Answer from the drawing. Dimensions are ordinates in mm from the lowest x, y and z of the part. Give positions to 0.01 mm unless a question says otherwise; leave off trailing zeros. Write each loop counter-clockwise with the first axis right and the second up, starting at its lowest first coordinate (ties: lowest second). Pieces come first, ordered by that corner, then holes. Notation, with made-up numbers: M 24,-5 L 77,-5 A30 cw 77,33 Z; hole C 9.5,42.5 d4. An arc over 180 degrees is marked long. Answer as a JSON object with one key per item and string values.
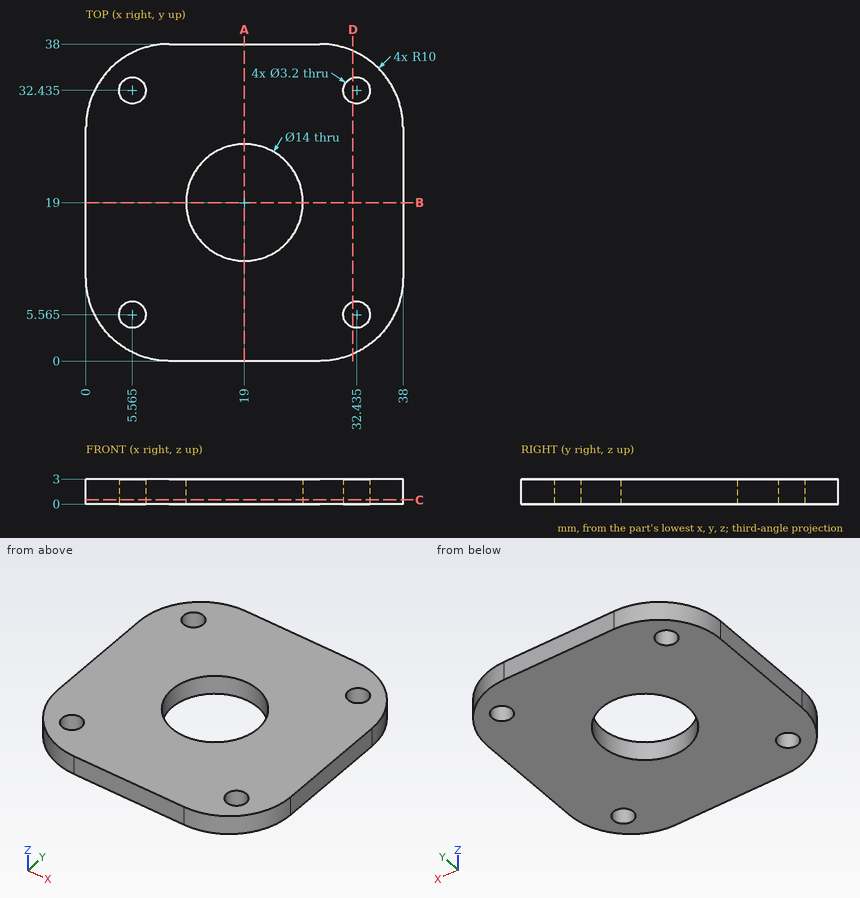
1. A cutting plane is placed at A-A, the plane x = 19. Give the vertices of the cut face in (y, z).
Verdict:
{"outline": "M 0,0 L 12,0 L 12,3 L 0,3 Z; M 26,0 L 38,0 L 38,3 L 26,3 Z"}
2. A cutting plane is placed at C-C, the plane z = 0.5. Give the vertices of the cut face in (x, y) (3 decimals), plus the area to 3 significant figures.
Verdict:
{"outline": "M 0,10 A10 ccw 10,0 L 28,0 A10 ccw 38,10 L 38,28 A10 ccw 28,38 L 10,38 A10 ccw 0,28 Z; hole C 5.565,5.565 d3.2; hole C 5.565,32.435 d3.2; hole C 19,19 d14; hole C 32.435,5.565 d3.2; hole C 32.435,32.435 d3.2", "area": "1,170 mm2"}
3. Consider line 1 along Y through (x, z) = (32, 1.05); line 2 along Y through (x, z) = (5, 0.9); line 3 along X through (y, z) = (6.5, 0.45). Determine where each line is inside the solid, lowest interval first.
Verdict:
{"line 1": "y = 0.83 to 4.03, 7.1 to 30.9, 33.97 to 37.17", "line 2": "y = 1.34 to 4.07, 7.06 to 30.94, 33.93 to 36.66", "line 3": "x = 0.63 to 4.27, 6.86 to 31.14, 33.73 to 37.37"}
4. A cutting plane is placed at D-D, the plane x = 32. Give the vertices of the cut face in (y, z).
Verdict:
{"outline": "M 0.83,0 L 4.03,0 L 4.03,3 L 0.83,3 Z; M 7.1,0 L 30.9,0 L 30.9,3 L 7.1,3 Z; M 33.97,0 L 37.17,0 L 37.17,3 L 33.97,3 Z"}
